The listing builds one solid part. Answer for the finished solid, in the listing's coordinates (mm). Face numbers are marked on the shaded views. A direction names the side the tool comes from. Coordinates: 2 decimals unless noted, no trailing zeros. Loops run counter-clockwise (first coordinate to the right, second up) from the corner with the lowest first, then second, coordinate; pieces in that order, holes last. Notation, with made-up numbers: (77.5, -37.75) - (115.5, -37.75) arc R10 ccw to (115.5, -29.75) - close; hole circle Ø2 at (2, 26.25). An arc over 180 degrees is marked (long way). Write each question's results on one line, items separated by ' | '. Start each with the question number.
(1) Given pin 1 Ø5 at (x, z) = (-9.9, 13.5) entering from +Y, flat-ended and moving along its own axis, determine where the tip first touches the part or whether it passes through.
(2) Find section A-A on x = 9.9. Determine the outline of the cut face in (y, z).
(3) Find section C-C on z = 4.95. Determine the outline of the cut face in (x, y).
(4) For the marked faces 1 and 2, determine the directions among +Z, -Z, +X, -X, +Y, -Y from which every point of the face is accessible in a straight line to the end or side of a thin tool.
(5) Find section B-B on z = -13.5. Determine the outline of the cut face in (x, y), then the cut area to 3 significant figures.
(6) Consider line 1 (X direction, y = 0.5, z = -13.5); line 2 (X direction, y = 0.6, z = 4.95); line 3 (Z direction, x = 3, y = 7.75). Determine where each line is inside the solid, lowest interval first. Write a range as from..to.
(7) Determine the mould class of the marked faces 3, 4 and 5 for opening direction Z: released by +Z, released by -Z, zero draft, split by the parting line, or undercut.
(8) Find section D-D on x = -9.9. Determine the outline of the cut face in (y, z), then the cut area to 3 significant figures.
from build123d import *

# Parameters (mm, degrees)
SKETCH_1_W          = 40
SKETCH_1_H          = 40.5
EXTRUDE_1_DEPTH     = 1.8
SKETCH_2_R          = 1.6
SKETCH_2_R_2        = 3
CUT_EXTRUDE_1_DEPTH = 2
SKETCH_3_W          = 40
SKETCH_3_H          = 9.8
EXTRUDE_2_DEPTH     = 1.8
SKETCH_4_R          = 1.15
CUT_EXTRUDE_2_DEPTH = 1.8


with BuildPart() as part:
    # 草图1 → 凸台-拉伸1 (new body)
    with BuildSketch(Plane(origin=(0, 0, 0), x_dir=(1, 0, 0), z_dir=(0, 1, 0))):
        Rectangle(SKETCH_1_W, SKETCH_1_H)
    extrude(amount=EXTRUDE_1_DEPTH)

    # 草图2 → 切除-拉伸1 (cut)
    with BuildSketch(Plane(origin=(0, 1.8, 0), x_dir=(1, 0, 0), z_dir=(0, 1, 0))):
        with Locations(Location((-9.9, 13.5, 0), (0, 0, 270))):
            Circle(SKETCH_2_R)
        with Locations(Location((0, 13.5, 0), (0, 0, 270))):
            Circle(SKETCH_2_R)
        with Locations(Location((9.9, 13.5, 0), (0, 0, 270))):
            Circle(SKETCH_2_R)
        with Locations(Location((0, 0, 0), (0, 0, 270))):
            Circle(SKETCH_2_R_2)
        with Locations(Location((9.9, 0, 0), (0, 0, 270))):
            Circle(SKETCH_2_R_2)
        with Locations(Location((-9.9, 0, 0), (0, 0, 270))):
            Circle(SKETCH_2_R_2)
        with Locations(Location((-9.9, -13.5, 0), (0, 0, 270))):
            Circle(SKETCH_2_R)
        with Locations(Location((0, -13.5, 0), (0, 0, 270))):
            Circle(SKETCH_2_R)
        with Locations(Location((9.9, -13.5, 0), (0, 0, 270))):
            Circle(SKETCH_2_R)
        with Locations(Location((-4.95, 4.949494924, 0), (0, 0, 270))):
            Circle(SKETCH_2_R)
        with Locations(Location((4.95, 4.949494924, 0), (0, 0, 270))):
            Circle(SKETCH_2_R)
        with Locations(Location((14.849494924, 4.95, 0), (0, 0, 270))):
            Circle(SKETCH_2_R)
        with Locations(Location((14.85, -4.949494924, 0), (0, 0, 270))):
            Circle(SKETCH_2_R)
        with Locations(Location((4.950505076, -4.95, 0), (0, 0, 270))):
            Circle(SKETCH_2_R)
        with Locations(Location((-4.950505076, -4.95, 0), (0, 0, 270))):
            Circle(SKETCH_2_R)
        with Locations(Location((-14.85, -4.949494924, 0), (0, 0, 270))):
            Circle(SKETCH_2_R)
        with Locations(Location((-14.849494924, 4.95, 0), (0, 0, 270))):
            Circle(SKETCH_2_R)
    extrude(amount=-CUT_EXTRUDE_1_DEPTH, mode=Mode.SUBTRACT)

    # 草图3 → 凸台-拉伸2 (add)
    with BuildSketch(Plane.XY.offset(20.25)):
        with Locations((0, 4.9)):
            Rectangle(SKETCH_3_W, SKETCH_3_H)
    extrude_2 = extrude(amount=EXTRUDE_2_DEPTH)

    # 草图4 → 切除-拉伸2 (cut)
    with BuildSketch(Plane.XY.offset(22.05)):
        with Locations((-17.5, 7.5)):
            Circle(SKETCH_4_R)
        with Locations((-2.5, 7.5)):
            Circle(SKETCH_4_R)
        with Locations((17.5, 7.5)):
            Circle(SKETCH_4_R)
        with Locations((-10.02, 8)):
            Circle(SKETCH_4_R)
        with BuildLine():
            Line((14.9, 9.8), (4.9, 9.8))
            ThreePointArc((4.9, 9.8), (9.9, 7.48038758), (14.9, 9.8))
        make_face()
    cut_extrude_2 = extrude(amount=-CUT_EXTRUDE_2_DEPTH, mode=Mode.SUBTRACT)

    # 镜向1: 凸台-拉伸2, 切除-拉伸2 across plane
    add(extrude_2.mirror(Plane.XY))
    add(cut_extrude_2.mirror(Plane.XY), mode=Mode.SUBTRACT)


solid = part.part
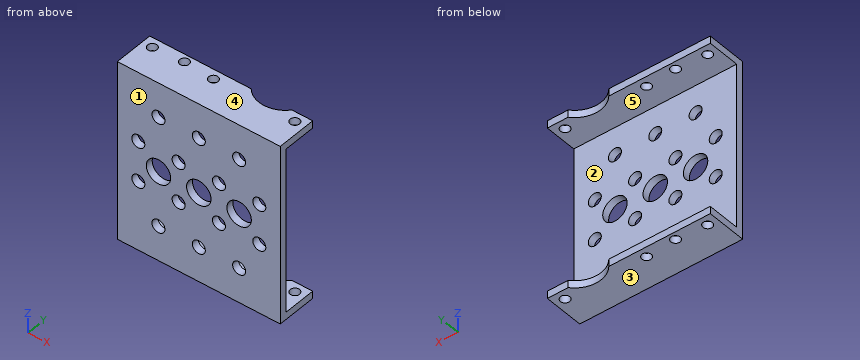
Values:
1) pin 1: stops at y = 1.8
2) outline: (0, -22.05) - (7.48, -22.05) - (7.48, -20.25) - (1.8, -20.25) - (1.8, -15.1) - (0, -15.1) - close; (0, -11.9) - (1.8, -11.9) - (1.8, -3) - (0, -3) - close; (0, 3) - (1.8, 3) - (1.8, 11.9) - (0, 11.9) - close; (0, 15.1) - (1.8, 15.1) - (1.8, 20.25) - (7.48, 20.25) - (7.48, 22.05) - (0, 22.05) - close
3) outline: (-20, 0) - (-16.45, 0) - (-16.45, 1.8) - (-20, 1.8) - close; (-13.25, 0) - (-6.55, 0) - (-6.55, 1.8) - (-13.25, 1.8) - close; (-3.35, 0) - (3.35, 0) - (3.35, 1.8) - (-3.35, 1.8) - close; (6.55, 0) - (13.25, 0) - (13.25, 1.8) - (6.55, 1.8) - close; (16.45, 0) - (20, 0) - (20, 1.8) - (16.45, 1.8) - close
4) face 1: +Z, -Z, +X, -X, -Y | face 2: +X, -X, +Y
5) outline: (-20, 0) - (-11.5, 0) - (-11.5, 1.8) - (-20, 1.8) - close; (-8.3, 0) - (-1.6, 0) - (-1.6, 1.8) - (-8.3, 1.8) - close; (1.6, 0) - (8.3, 0) - (8.3, 1.8) - (1.6, 1.8) - close; (11.5, 0) - (20, 0) - (20, 1.8) - (11.5, 1.8) - close | area: 54.7 mm²
6) line 1: x = -20..-11.5, -8.3..-1.6, 1.6..8.3, 11.5..20 | line 2: x = -20..-16.45, -13.25..-6.55, -3.35..3.35, 6.55..13.25, 16.45..20 | line 3: z = -22.05..-20.25, 20.25..22.05
7) face 3: released by -Z | face 4: released by +Z | face 5: undercut
8) outline: (0, -22.05) - (6.86, -22.05) - (6.86, -20.25) - (1.8, -20.25) - (1.8, -15.1) - (0, -15.1) - close; (0, -11.9) - (1.8, -11.9) - (1.8, -3) - (0, -3) - close; (0, 3) - (1.8, 3) - (1.8, 11.9) - (0, 11.9) - close; (0, 15.1) - (1.8, 15.1) - (1.8, 20.25) - (6.86, 20.25) - (6.86, 22.05) - (0, 22.05) - close; (9.14, -22.05) - (9.8, -22.05) - (9.8, -20.25) - (9.14, -20.25) - close; (9.14, 20.25) - (9.8, 20.25) - (9.8, 22.05) - (9.14, 22.05) - close | area: 77.6 mm²
